Could you check a few things on this model? Use its own coordinates, in mm. A direction names the side the tool comes from. Coordinates: 2 decimals unless noted, no trailing zeros. Write each loop counter-clockwise with the first axis right and the second up, starting at its lowest first coordinate (ties: lowest second). Pieces come first, ordered by that corner, then holes. Notation, with made-up numbers: (10.25, -21) - (33.25, -21) arc R13 ccw to (33.25, -16) - close; hole circle Ø2 at (66.5, 35). An arc over 180 degrees is marked (long way). Write item = value, one per line. Start each with the question number.
Autodesk Fusion 360 part; units mm, degrees
sketch "Sketch1" plane through (0, 0, 0) normal (0, 0, 1) x (1, 0, 0)
  circle A0 centre (0, 0) radius 5
  circle A1 centre (0, 0) radius 10
  dimension "d1" = 10
  dimension "d2" = 20
extrude "Extrude1" add sketch "Sketch1" along normal blind 7.5
sketch "Sketch2" plane through (0, 0, 0) normal (0, 0, 1) x (1, 0, 0)
  circle A0 centre (0, 0) radius 3.05
  circle A1 centre (0, 0) radius 7.5
  dimension "d5" = 6.1
  dimension "d6" = 15
extrude "Extrude2" add sketch "Sketch2" against normal blind 10
sketch "草图3" plane through (0, 0, 0) normal (0, 0, 1) x (1, 0, 0)
  circle A0 centre (0, 0) radius 6
  dimension "d9" = 12
extrude "拉伸3" cut sketch "草图3" along normal blind 8
sketch "草图4" plane through (0, 0, 0) normal (0, 0, 1) x (1, 0, 0)
  circle A0 centre (0, 0) radius 3.25
  dimension "d12" = 6.5
extrude "拉伸4" cut sketch "草图4" against normal blind 10
sketch "草图5" plane through (0, 0, 0) normal (0, 0, 1) x (1, 0, 0)
  circle A0 centre (0, 0) radius 5.75
  circle A1 centre (0, 0) radius 6
  dimension "d15" = 11.5
extrude "拉伸5" add sketch "草图5" along normal blind 7.5
sketch "草图6" plane through (0, 0, 0) normal (0, 0, 1) x (1, 0, 0)
  circle A0 centre (0, 0) radius 5.4
  circle A1 centre (0, 0) radius 5.75
  dimension "d18" = 10.8
  dimension "d19" = 11.5
extrude "拉伸6" add sketch "草图6" along normal blind 7.5
sketch "草图7" plane through (0, 0, 7.5) normal (0, 0, 1) x (-1, 0, 0)
  circle A0 centre (0, 0) radius 5.4
  circle A1 centre (0, 0) radius 10
extrude "拉伸7" add sketch "草图7" against normal blind 7 contours A0
sketch "草图8" plane through (0, 0, 7.5) normal (0, 0, 1) x (-1, 0, 0)
  circle A0 centre (0, 0) radius 10
  circle A1 centre (0, 0) radius 5.3
  dimension "d24" = 10.6
extrude "拉伸8" cut sketch "草图8" against normal blind 7 contours A1
1) If I drill on probe 1 along Y at (x, z) = (0, -3.25); probe 2 along Y at (x, z) = (0, 6.25); probe 3 along Z at (x, y) = (-0.25, -4.5), over which ranges is the centre line in solid material (lowest first)? Write a range as [from, to].
2) Which directions (+Z, -Z, +X, -X, +Y, -Y) give clear straight access to the entire face, cutting with the end or side of a thin tool? Please do faces 4 (the cylindrical face through (-1.17, 5.27, 0.25)), 5 (the flat face through (2, -3, -10)), 6 (the flat face through (4, 7, 0)).
3) Thinking about a two-plate mould opening in X: for faces 1 (the cylindrical face through (-7.493, 0.33, -4.93)), 2 (the cylindrical face through (-4.896, 2.03, 4.049)), 3 (the flat face through (-4, 4, 7.5)), which applies, +X half, -X half, draft (parallel to the pull), parting line (faces both ways), or undercut?
4) Suppose I cut it at C-C on z = -3.5. Please give me the cut outline in (x, y).
5) For P1, Ø5, axis at x = -1, z = -6.5, coming from the +Y side; P2, Ø8.5, axis at x = 0, y = 0, coming from the -Z side; P3, Ø6, axis at y = -7.5, z = 3, coming from the -X side; P4, Ø1.5, axis at y = -6.5, z = 5, coming from the +X side, each with a flat end and sliding along its axis, tell me the tip position at first contact or that it passes through.
6) Suppose I cut it at D-D on y = -3.75. Please give me the cut outline in (x, z).
7) Suppose I cut it at A-A on x = 0. Please give me the cut outline in (y, z).
Reply:
q1.probe_1 = [-7.5, -3.25], [3.25, 7.5]
q1.probe_2 = [-10, -5.3], [5.3, 10]
q1.probe_3 = [-10, 0]
q2.face_4 = none
q2.face_5 = -Z, +X, -X, +Y, -Y
q2.face_6 = -Z
q3.face_1 = parting line
q3.face_2 = undercut
q3.face_3 = draft
q4.outline = circle Ø15 at (0, 0); hole circle Ø6.5 at (0, 0)
q5.P1 = 7.5
q5.P2 = -10
q5.P3 = -8.93
q5.P4 = 8.18
q6.outline = (-9.27, 0) - (-6.5, 0) - (-6.5, -10) - (6.5, -10) - (6.5, 0) - (9.27, 0) - (9.27, 7.5) - (3.75, 7.5) - (3.75, 0.5) - (3.89, 0.5) - (3.89, 0) - (-3.89, 0) - (-3.89, 0.5) - (-3.75, 0.5) - (-3.75, 7.5) - (-9.27, 7.5) - close
q7.outline = (-10, 0) - (-7.5, 0) - (-7.5, -10) - (-3.25, -10) - (-3.25, 0) - (-5.4, 0) - (-5.4, 0.5) - (-5.3, 0.5) - (-5.3, 7.5) - (-10, 7.5) - close; (3.25, -10) - (7.5, -10) - (7.5, 0) - (10, 0) - (10, 7.5) - (5.3, 7.5) - (5.3, 0.5) - (5.4, 0.5) - (5.4, 0) - (3.25, 0) - close
